```python
from build123d import *

# Parameters (mm, degrees)
SKETCH1_W               = 25.4
SKETCH1_H               = 25.4
SKETCH1_W_2             = 19.05
SKETCH1_H_2             = 19.05
EXTRUDE1_DEPTH          = 609.6
F_1_4_CLEARANCE_HOLE1_D = 6.7564
F_1_4_CLEARANCE_HOLE2_D = 6.7564
LPATTERN1_COUNT         = 18
LPATTERN1_PITCH         = 27.94


with BuildPart() as part:
    # Sketch1 → Extrude1 (new body)
    with BuildSketch(Plane.XY):
        Rectangle(SKETCH1_W, SKETCH1_H)
        Rectangle(SKETCH1_W_2, SKETCH1_H_2, mode=Mode.SUBTRACT)
    extrude(amount=-EXTRUDE1_DEPTH)

    # 1/4 Clearance Hole1 (through all)
    with Locations(Plane(origin=(0, 12.7, 0), x_dir=(-1, 0, 0), z_dir=(0, 1, 0))):
        with Locations((0, -584.2)):
            Hole(F_1_4_CLEARANCE_HOLE1_D / 2)

    # 1/4 Clearance Hole2 (through all)
    with Locations(Plane(origin=(0, 12.7, 0), x_dir=(-1, 0, 0), z_dir=(0, 1, 0))):
        with Locations((0, -508)):
            f_1_4_clearance_hole2 = Hole(F_1_4_CLEARANCE_HOLE2_D / 2)

    # LPattern1: 1/4 Clearance Hole2 ×18
    with Locations(*[(0, 0, i * LPATTERN1_PITCH) for i in range(1, LPATTERN1_COUNT)]):
        add(f_1_4_clearance_hole2, mode=Mode.SUBTRACT)


solid = part.part
```
Input: part model. Units: mm. Frame: model coordinates. A direction names the side the tool comes from. Give positions to 0.01 mm unless a question says otherwise; leave off trailing zeros. Order: outer loops, then holes, each group sorted by start corner. A loop starts at its lowest first (then second) coordinate and runs counter-clockwise, first axis right, second up.
1. Line query: probe 1 along Y at (x, z) = (6.75, -203.5) (3 decimals); probe 2 along X at (y, z) = (-11.65, -284.48). Output: solid intervals per line, ascending.
Computed:
probe 1: y = -12.7 to -9.525, 9.525 to 12.7
probe 2: x = -12.7 to -3.38, 3.38 to 12.7
2. Set-up query: faces 1 (the face through (-9.525, 0, -301)), 2 (the face through (11, 0, 0)). Return all of +Z, -Z, +X, -X, +Y, -Y with unobstructed straight access to the full face (end or side cutting, diameter ignored); none if empty.
Computed:
face 1: +Z, -Z
face 2: +Z, +X, -X, +Y, -Y
3. Pin query (flat end, axial travel): pin 1 Ø11 at (x, z) = (0, -116.84) entering from +Y; pin 2 Ø4 at (x, z) = (0, -340.36) entering from +Y. Return the tip coordinate at first contact, or that it passes through.
Computed:
pin 1: stops at y = 12.7
pin 2: passes through
4. Draft query along X for faces 3 (the face through (0, 9.525, -301)), 4 (the face through (11, 0, -609.6)), 5 (the face through (-12.7, 0, -301)). Return one class per face: released by +X, released by -X, zero draft, split by the parting line, or undercut.
Computed:
face 3: undercut
face 4: zero draft
face 5: released by -X
5. Cut plane A-A (y = 0.75). Return loops of the section in (x, z) (3 decimals), and give its area (3 significant figures).
Computed:
outline: (-12.7, -609.6) - (-9.525, -609.6) - (-9.525, 0) - (-12.7, 0) - close; (9.525, -609.6) - (12.7, -609.6) - (12.7, 0) - (9.525, 0) - close
area: 3,870 mm2
